The model under review builds one solid part; all positions refer to its coordinate system, in mm. Face numbers are marked on the shaded views. A direction names the side the tool comes from. Coordinates: 2 decimals unless noted, no trailing zeros. Order: outer loops, then holes, each group sorted by start corner. A loop starts at its lowest first (then second) coordinate and runs counter-clockwise, first axis right, second up. Notation, with made-up numbers: M -22.75,32 L 19.25,32 A26 cw 19.25,48 Z; hole C -29,86.25 d4. An arc over 180 degrees is marked long. Answer in a Markdown table with one row per item.
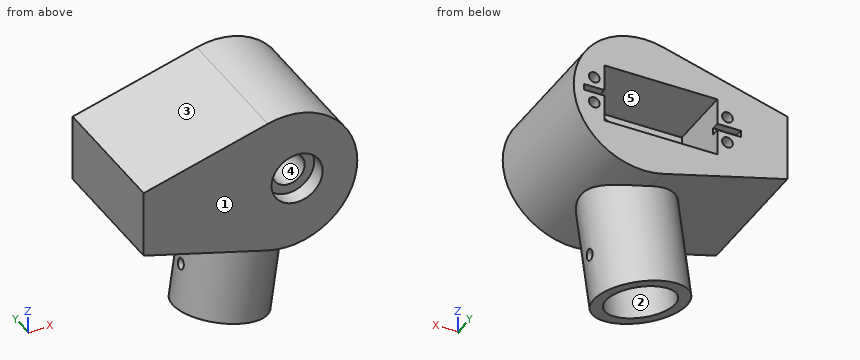
from build123d import *

# Parameters (mm, degrees)
BOSS_EXTRUDE1_DEPTH       = 40
SKETCH2_W                 = 33.6
SKETCH2_H                 = 17.6
CUT_EXTRUDE1_DEPTH        = 20
SKETCH3_W                 = 7
SKETCH3_H                 = 2
CUT_EXTRUDE2_DEPTH        = 2.4
SKETCH4_W                 = 7
SKETCH4_H                 = 1.8
CUT_EXTRUDE3_DEPTH        = 2.4
REVOLVE1_START            = -44.95139953
REVOLVE1_OUTLINE_R        = 13.5
REVOLVE1_DEPTH            = 30.829897511
M18_CLEARANCE_HOLE1_D     = 20
M18_CLEARANCE_HOLE1_DEPTH = 25
SKETCH9_W                 = 1.6
SKETCH9_H                 = 27
CUT_EXTRUDE4_DEPTH        = 76.299241718
CUT_EXTRUDE4_DEPTH_BACK   = 76.299241718
SKETCH18_R                = 1.6
SCALE2_SCALE              = 1.25
SKETCH20_R                = 9.5
CUT_EXTRUDE5_DEPTH        = 5
SKETCH21_R                = 6
CUT_EXTRUDE6_DEPTH        = 87.235197147
CUT_EXTRUDE8_START        = -6
SKETCH25_R                = 9.5
CUT_EXTRUDE8_DEPTH        = 6
SKETCH27_R                = 2
CUT_EXTRUDE9_DEPTH        = 12


with BuildPart() as part:
    # Sketch1 → Boss-Extrude1 (new body)
    with BuildSketch(Plane(origin=(0, 40, 0), x_dir=(1, 0, 0), z_dir=(0, 1, 0))):
        with BuildLine():
            Line((-5.61521172, 20.235350191), (-42.5, 10))
            Line((-42.5, 10), (-42.5, -10))
            Line((-42.5, -10), (-5.61521172, -20.235350191))
            ThreePointArc((-5.61521172, -20.235350191), (21, 0), (-5.61521172, 20.235350191))
        make_face()
    extrude(amount=-BOSS_EXTRUDE1_DEPTH)

    # Sketch2 → Cut-Extrude1 (cut)
    with BuildSketch(Plane(origin=(0, 40, 0), x_dir=(-1, 0, 0), z_dir=(0, 1, 0))):
        with Locations((4.9, 0)):
            Rectangle(SKETCH2_W, SKETCH2_H)
    extrude(amount=-CUT_EXTRUDE1_DEPTH, mode=Mode.SUBTRACT)

    # Sketch3 → Cut-Extrude2 (cut)
    with BuildSketch(Plane(origin=(0, 40, 0), x_dir=(-1, 0, 0), z_dir=(0, 1, 0))):
        with Locations((25.2, 0)):
            Rectangle(SKETCH3_W, SKETCH3_H)
    extrude(amount=-CUT_EXTRUDE2_DEPTH, mode=Mode.SUBTRACT)

    # Sketch4 → Cut-Extrude3 (cut)
    with BuildSketch(Plane(origin=(0, 40, 0), x_dir=(-1, 0, 0), z_dir=(0, 1, 0))):
        with Locations((-14.5, 0)):
            Rectangle(SKETCH4_W, SKETCH4_H)
    extrude(amount=-CUT_EXTRUDE3_DEPTH, mode=Mode.SUBTRACT)

    # Revolve1: read off the stored shape, not the designer's step
    # Revolve1 outline → Revolve1 (add)
    with BuildSketch(Plane(origin=(0, 0, 0), x_dir=(0.9799247046208294, -0.02083962380947531, -0.19827577601224947), z_dir=(0.19936793441719802, 0.10243002349202102, 0.9745565745577031)).offset(REVOLVE1_START)):
        with Locations((-1.9070974, 22.005607966)):
            Circle(REVOLVE1_OUTLINE_R)
    extrude(amount=REVOLVE1_DEPTH)

    # M18 Clearance Hole1
    with Locations(Plane(origin=(-8.961867673, -4.60437291, -43.807681948), x_dir=(-0.9799247046208296, 0.02083962380947534, 0.19827577601224922), z_dir=(-0.19936793441719777, -0.10243002349202121, -0.9745565745577032))):
        with Locations((1.9070974, 22.005607966)):
            Hole(M18_CLEARANCE_HOLE1_D / 2, depth=M18_CLEARANCE_HOLE1_DEPTH)

    # Sketch9 → M3.5 Clearance Hole1 (revolve, cut)
    with BuildSketch(Plane(origin=(-18.009225855, 18.806465846, -31.591069121), x_dir=(-0.12392681772022805, 0.7153744254872676, -0.6876638533531477), z_dir=(0.1561720753640579, 0.6984304843277114, 0.6984304843277114))):
        with Locations((0.8, 13.5)):
            Rectangle(SKETCH9_W, SKETCH9_H)
    revolve(axis=Axis((-11.78670398, 18.674134235, -32.850120299), (-0.9799247046208297, 0.020839623809475325, 0.19827577601224802)), mode=Mode.SUBTRACT)

    # Sketch18 → Cut-Extrude4 (cut, two sides: drawn at the far end of the back side and taken through both)
    with BuildSketch(Plane(origin=(-1.740210315, 0.03700828, 0.352110268), x_dir=(-0.19823095447813932, 0.004215689735382395, -0.9801462730872066), z_dir=(0.9799247046208297, -0.020839623809475356, -0.19827577601224802)).offset(-CUT_EXTRUDE4_DEPTH_BACK)):
        with Locations(Location((34.613136918, 18.419306886, 0), (0, 0, 359.758405588))):
            Circle(SKETCH18_R)
    extrude(amount=CUT_EXTRUDE4_DEPTH + CUT_EXTRUDE4_DEPTH_BACK, mode=Mode.SUBTRACT)


with BuildPart() as part_1:
    # Scale2: scaled about (0, 0, 0)
    add(part.part.scale(SCALE2_SCALE))

    # Sketch20 → Cut-Extrude5 (cut)
    with BuildSketch(Plane(origin=(0, 25, 0), x_dir=(1, 0, 0), z_dir=(0, 1, 0))):
        with Locations(Location((3.875, 0, 0), (0, 0, 270))):
            Circle(SKETCH20_R)
    extrude(amount=-CUT_EXTRUDE5_DEPTH, mode=Mode.SUBTRACT)

    # Sketch21 → Cut-Extrude6 (cut, through all)
    with BuildSketch(Plane(origin=(0, 20, 0), x_dir=(1, 0, 0), z_dir=(0, 1, 0))):
        with Locations(Location((3.875, 0, 0), (0, 0, 270))):
            Circle(SKETCH21_R)
    extrude(amount=-CUT_EXTRUDE6_DEPTH, mode=Mode.SUBTRACT)

    # Sketch25 → Cut-Extrude8 (cut)
    with BuildSketch(Plane.XZ.offset(CUT_EXTRUDE8_START)):
        with Locations(Location((3.875, 0, 0), (0, 0, 90))):
            Circle(SKETCH25_R)
    extrude(amount=CUT_EXTRUDE8_DEPTH, mode=Mode.SUBTRACT)

    # Sketch27 → Cut-Extrude9 (cut)
    with BuildSketch(Plane(origin=(0, 50, 0), x_dir=(1, 0, 0), z_dir=(0, 1, 0))):
        with Locations(Location((18.625, 5, 0), (0, 0, 270))):
            Circle(SKETCH27_R)
        with Locations(Location((18.625, -5, 0), (0, 0, 270))):
            Circle(SKETCH27_R)
        with Locations(Location((-30.875, 5, 0), (0, 0, 270))):
            Circle(SKETCH27_R)
        with Locations(Location((-30.875, -5, 0), (0, 0, 270))):
            Circle(SKETCH27_R)
    extrude(amount=-CUT_EXTRUDE9_DEPTH, mode=Mode.SUBTRACT)


solid = part_1.part
(1) The part is to be moulded in two halves that separate along X. For the marked faces 1, 2 and 3, say which applies: +X half, -X half, draft (parallel to the pull), parting line (faces both ways), or undercut.
Report:
| item | result |
|---|---|
| face 1 | draft |
| face 2 | undercut |
| face 3 | -X half |
(2) Take a section at C-C (x = 0). State how many separate pieces and enclosed holes the cut face has, then the cut area to 3 significant figures.
Report:
| item | result |
|---|---|
| separate pieces | 2 |
| enclosed holes | 1 |
| area | 2,280 mm^2 |
(3) Machinability: for the marked faces 4 and 5, which of the approach directions +Z, -Z, +X, -X, +Y, -Y give a long, thin tool a straight path to every point of the face, cutting with its end or side? Answer none if there is none.
Report:
| item | result |
|---|---|
| face 4 | +Y, -Y |
| face 5 | +Y |
(4) Take a section at A-A (z = 0). Write out the cut boundary in (x, y) (3 decimals).
Report:
| item | result |
|---|---|
| outline | M -53.125,0 L -5.625,0 L -5.625,6 L -2.125,6 L -2.125,20 L -5.625,20 L -5.625,25 L -27.125,25 L -27.125,47 L -35.875,47 L -35.875,50 L -53.125,50 Z; M 9.875,6 L 13.375,6 L 13.375,0 L 26.25,0 L 26.25,50 L 22.5,50 L 22.5,47 L 14.875,47 L 14.875,25 L 13.375,25 L 13.375,20 L 9.875,20 Z |
(5) Take a section at D-D (z = -17). Write out the cut boundary in (x, y), then the cut area to 3 significant figures.
Report:
| item | result |
|---|---|
| outline | M -36.91,0 L 20,0 L 20,50 L -36.91,50 Z |
| area | 2,850 mm^2 |
(6) To check wall thickness, follow line 1 (X direction, y = 13, z = 0) (3 decimals); line 2 (Z direction, x = -29.5, y = 41); line 3 (X direction, y = 44, z = -5) (3 decimals). State the ranges of each line that lie inside material, in increasing order. Write a range as [from, to].
Report:
| item | result |
|---|---|
| line 1 | [-53.125, -2.125], [9.875, 26.25] |
| line 2 | [-19.06, -6.45], [-3.55, 3.55], [6.45, 19.06] |
| line 3 | [-53.125, -32.875], [-28.875, -27.125], [14.875, 16.625], [20.625, 25.769] |
(7) Insertion check: P1, Ø3, axis at x = -29, y = 15.5, coming from the +Z side; P2, Ø2.5, axis at x = -31.5, y = 48.5, coming from the -Z side; P3, Ø3.5, axis at x = -31.5, y = 49, coming from the +Z side. Each pin has a flat end and moves straight along its axis. Give the tip position at first contact, or say it passes through.
Report:
| item | result |
|---|---|
| P1 | z = 19.61 |
| P2 | z = -18.85 |
| P3 | z = 18.99 |
(8) Take a section at B-B (x = -34). Write out the cut boundary in (y, z).
Report:
| item | result |
|---|---|
| outline | M 0,-17.81 L 50,-17.81 L 50,-1.25 L 47,-1.25 L 47,1.25 L 50,1.25 L 50,17.81 L 0,17.81 Z |
